The model under review builds one solid part; all positions refer to its coordinate system, in mm. Face numbers are marked on the shaded views. A direction names the side the tool comes from. Coordinates: 2 decimals unless noted, no trailing zeros. Order: outer loops, then holes, each group sorted by start corner. A loop starts at its lowest first (then second) coordinate and runs counter-clockwise, first axis right, second up.
Autodesk Inventor part; units mm, degrees
ref_plane "WorkPlane12" through (0, 0, 0) normal (0, 0, 1) x (1, 0, 0)
ref_plane "MSC_PF1" through (0, 0, 0) normal (1, 0, 0) x (0, 1, 0)
ref_plane "MSC_PT1" through (0, 0, 0) normal (0, 0, -1) x (-1, 0, 0)
ref_plane "WorkPlane12" through (0, 0, 0) normal (0, 0, 1) x (1, 0, 0)
sketch "Boceto1" plane through (0, 0, 0) normal (0, 0, 1) x (1, 0, 0)
  point P0 (0, 0)
sketch "Boceto2" plane through (0, 0, 0) normal (0, 0, 1) x (1, 0, 0)
  circle A0 centre (0, 0) radius 2.5
  dimension "d1" = 5
extrude "Extrusión1" add sketch "Boceto2" against normal blind 25
chamfer "Chaflán1" distance 0.4 angle 45 1 edges at (-2.5, 0, -25)
sketch "Boceto3" plane through (0, 0, 0) normal (0, 0, 1) x (1, 0, 0)
  circle A0 centre (0, 0) radius 3.15
  circle A1 centre (0, 0) radius 2.5 construction
  dimension "d7" = 6.3
extrude "Extrusión2" add sketch "Boceto3" along normal blind 5.6
sketch "Boceto4" plane through (0, 0, 0) normal (0, 1, 0) x (-1, 0, 0)
  line L0 (0, 0) -> (5.1754, 0)
  line L1 (0, 3.5167) -> (0, 0)
  line L2 (5.3971, 1) -> (0, 3.5167)
  line L3 (0, -0.8101) -> (0, 4.2379)
  line L4 (-2.5, 0) -> (2.5, 0)
  arc A0 (5.1754, 0) -> (5.3971, 1) centre (5.1754, 0.5246) ccw
  dimension "d14" = 25
  dimension "d16" = 1
  dimension "d45" = 5.7
revolve "Revolución1" add sketch "Boceto4" angle 360 about axis through (0, 0, 3.5167) along (0, 0, -1)
fillet "Empalme1" radius 0.2994 1 edges at (-2.5, 0, 0)
sketch "Boceto5" plane through (0, 0, 5.6) normal (0, 0, 1) x (1, 0, 0)
  line L0 (-3.5, 2.0207) -> (-3.5, -2.0207)
  line L1 (0, 4.0415) -> (-3.5, 2.0207)
  line L2 (3.5, 2.0207) -> (0, 4.0415)
  line L3 (3.5, -2.0207) -> (3.5, 2.0207)
  line L4 (0, -4.0415) -> (3.5, -2.0207)
  line L5 (-3.5, -2.0207) -> (0, -4.0415)
  circle A0 centre (0, 0) radius 3.5 construction
  circle A1 centre (0, 0) radius 3.15 construction
  dimension "d20" = 7
  dimension "d35" = 120
  dimension "d36" = 120
extrude "Extrusión3" add sketch "Boceto5" against normal blind 5.6
sketch "Boceto9" plane through (0, 0, 0) normal (1, 0, 0) x (0, 1, 0)
  line L0 (-4.0415, 5.6) -> (-4.0415, 5.2874)
  line L1 (-4.0415, 5.2874) -> (-3.5, 5.6)
  line L2 (-3.5, 5.6) -> (-4.0415, 5.6)
  line L3 (-4.0415, 5.6) -> (-4.0415, 1.6322)
  line L4 (-4.0415, 5.6) -> (-2.0207, 5.6)
  line L5 (0, -1.12) -> (0, 6.72)
  dimension "d28" = 30
  dimension "d29" = 3.5
revolve "Revolución2" cut sketch "Boceto9" angle 360 about axis through (0, 0, -10) along (0, 0, 1)
thread "Rosca1"
ref_plane "MSC_PF1" through (0, 0, 0) normal (1, 0, 0) x (0, 1, 0)
ref_plane "MSC_PT1" through (0, 0, 0) normal (0, 0, -1) x (-1, 0, 0)
equation "\"d2\" = NLG"
equation "\"d4\" = msp_z"
equation "\"d5\" = msp_z"
equation "\"d7\" = 0.9 * Smax"
equation "\"d8\" = Kmax"
equation "\"d18\" = msp_r"
equation "\"d20\" = Smax"
equation "\"d21\" = Kmax"
equation "\"d33\" = B"
equation "\"d1\" = NND"
equation "\"d16\" = Cmin"
equation "\"d45\" = 0.5 * Dcmax"
equation "\"d29\" = 0.5 * Smax"
equation "\"NND\" = 5"
equation "\"NLG\" = 25"
equation "\"PTC\" = 0.8"
equation "\"msp_z\" = 0.5 * PTC"
equation "\"Smax\" = 7"
equation "\"Kmax\" = 5.6"
equation "\"Dcmax\" = 11.4"
equation "\"Cmin\" = 1"
equation "\"msp_r\" = 0.0598802 * NND"
equation "\"B\" = 16"
equation "\"THREADDIA\" = NND"
properties part number "ANSI B18.2.3.4M - M5 x 0.8x25" material "Acero, suave"
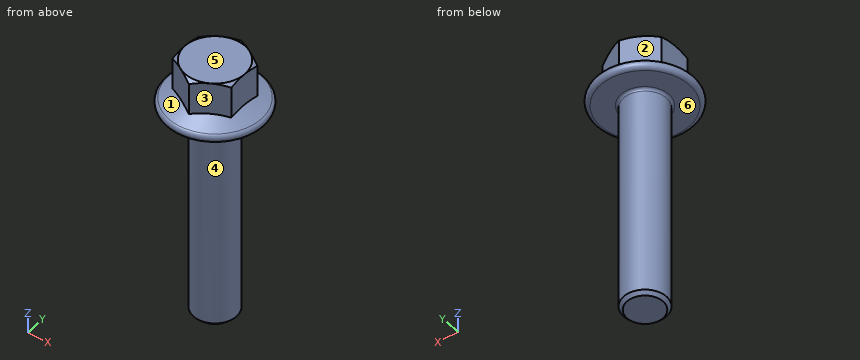
(1) Consider section A-A (z = -8). Give the boundary of the cut face in (x, y).
(2) Tool access review of the marked faces 1, 2 and 3: name each direction out of +Z, -Z, +X, -X, +Y, -Y from which nothing blocks a thin tool from reaching the whole face with its end or side.
(3) Insertion check: pin 1 Ø1.5 at (x, y) = (-3.5, -3) entering from +Z; pin 2 Ø1.2 at (y, z) = (-0.5, 4) entering from -X; pin 3 Ø1 at (x, z) = (2, 2) entering from +Y. Each pin has a flat end and moves straight along its axis. Give the tip position at first contact, or say it passes through.
(4) The part is to be moulded in two halves that separate along Z. For the marked faces 4, 5 and 6, say which applies: +Z half, -Z half, draft (parallel to the pull), parting line (faces both ways), or undercut.
(5) Wall thickness on line 1 (X direction, y = -1.25, z = 4); line 2 (Z direction, x = -2, y = 2); line 3 (X direction, y = -2, z = -12): over which ranges is each line inside the solid? List them lowest first.
Findings:
1. outline: circle Ø5 at (0, 0)
2. face 1: +Z
2. face 2: +Z, -X, +Y
2. face 3: +Z, +X, -Y
3. pin 1: stops at z = 1.72
3. pin 2: stops at x = -3.5
3. pin 3: stops at y = 3.86
4. face 4: draft
4. face 5: +Z half
4. face 6: -Z half
5. line 1: x = -3.5 to 3.5
5. line 2: z = 0 to 5.6
5. line 3: x = -1.5 to 1.5
